from build123d import *

# Parameters (mm, degrees)
F0_W      = 28
F0_H      = 20
F1_DEPTH  = 20
F3_DEPTH  = 20
F6_DEPTH  = 17.5
F7_W      = 1.5
F7_H      = 4
F8_DEPTH  = 40
F12_DEPTH = 15
F15_D     = 14.5
F17_DEPTH = 20
F19_DEPTH = 12.5


with BuildPart() as f1:
    # F0 (on Top) → F1 (new body)
    with BuildSketch(Plane.XY):
        Rectangle(F0_W, F0_H)
    extrude(amount=F1_DEPTH)


with BuildPart() as f3:
    # F2 (on Top) → F3 (new body)
    with BuildSketch(Plane.XY):
        Polygon((-14, 3.5), (-7.5, 10), (-14, 10), align=None)
    extrude(amount=F3_DEPTH)


with BuildPart() as f4_1:
    # F4: instance of F3
    add(f3.part.mirror(Plane.YZ))


with BuildPart() as f6:
    # F5 (on Right) → F6 (new body, symmetric)
    with BuildSketch(Plane.YZ):
        Polygon((-4.741189, 25.532488), (10, 0), (10, 25.532488), align=None)
    extrude(amount=F6_DEPTH, both=True)


with BuildPart() as f8:
    # F7 (on Top) → F8 (new body)
    with BuildSketch(Plane.XY):
        with Locations((-13.25, 0)):
            Rectangle(F7_W, F7_H)
    extrude(amount=F8_DEPTH)


with BuildPart() as f9_1:
    # F9: instance of F8
    add(f8.part.mirror(Plane.YZ))


with BuildPart() as f1_1:
    add(f1.part)

    # F10: cut F3, F4_1, F6, F8, F9_1
    add(f3.part, mode=Mode.SUBTRACT)
    add(f4_1.part, mode=Mode.SUBTRACT)
    add(f6.part, mode=Mode.SUBTRACT)
    add(f8.part, mode=Mode.SUBTRACT)
    add(f9_1.part, mode=Mode.SUBTRACT)


with BuildPart() as f12:
    # F11 (on Right) → F12 (new body, symmetric)
    with BuildSketch(Plane.YZ):
        Polygon((-10, 24.094011), (-10, 1), (0, 6.773503), align=None)
    extrude(amount=F12_DEPTH, both=True)


with BuildPart() as f1_2:
    add(f1_1.part)

    # F13: cut F12
    add(f12.part, mode=Mode.SUBTRACT)

    # F15 (through all)
    with Locations(Plane(origin=(0, 2.933013, 1.693376), x_dir=(1, 0, 0), z_dir=(0, -0.866025, -0.5))):
        with Locations((0, 15.116025)):
            Hole(F15_D / 2)


with BuildPart() as f17:
    # F16 (on Right) → F17 (new body, symmetric)
    with BuildSketch(Plane.YZ):
        Polygon((-7.5, 13.205771), (6, 21), (-12, 21), align=None)
    extrude(amount=F17_DEPTH, both=True)


with BuildPart() as f19:
    # F18 (on face) → F19 (new body, symmetric)
    with BuildSketch(Plane(origin=(0, 7.5, 4.330127), x_dir=(-1, 0, 0), z_dir=(0, 0.866025, 0.5))):
        Polygon((14, 17.490759), (8, 17.490759), (14, 8), align=None)
    extrude(amount=F19_DEPTH, both=True)


with BuildPart() as f20_1:
    # F20: instance of F19
    add(f19.part.mirror(Plane.YZ))


with BuildPart() as f1_3:
    add(f1_2.part)

    # F21: cut F20_1, F19, F17
    add(f20_1.part, mode=Mode.SUBTRACT)
    add(f19.part, mode=Mode.SUBTRACT)
    add(f17.part, mode=Mode.SUBTRACT)


solid = f1_3.part
Verification items for the finished model (mm, model axes). A direction names the side the tool comes from. Coordinates: 2 decimals unless noted, no trailing zeros. Write each loop counter-clockwise with the first axis right and the second up, starting at its lowest first coordinate (ties: lowest second). Pieces come first, ordered by that corner, then holes. Notation, with made-up numbers: M 71,44 L 125,44 A17 ccw 125,74 Z; hole C -7,-39 d11. An arc over 180 degrees is marked long. One line per question, with ' | ' between items.
1) Sectioned sample at D-D on x = 5.5. Record the cut outline in (y, z).
Solutions:
outline: M -10,0 L 10,0 L 2.3,13.33 L -2.26,10.69 L 0,6.77 L -10,1 Z
2) Sectioned sample at B-B on z = 2.5. Record the cut outline in (x, y), then the cut area to 3 significant figures.
Solutions:
outline: M -14,-7.4 L 14,-7.4 L 14,-2 L 12.5,-2 L 12.5,2 L 14,2 L 14,3.5 L 8.94,8.56 L -8.94,8.56 L -14,3.5 L -14,2 L -12.5,2 L -12.5,-2 L -14,-2 Z | area: 409 mm^2
3) Depth check by flat-ended pin: pin 1 Ø1.5 at (y, z) = (7.5, 5) entering from +X; pin 2 Ø1 at (x, z) = (-10.5, 3.5) entering from +Y; pin 3 Ø8 at (x, y) = (10, 7.5) entering from +Z; pin 4 Ø4 at (y, z) = (-6, 4.5) entering from +X. Enter the tip coordinate at first touch or a pass-through.
Solutions:
pin 1: x = 10.75 | pin 2: y = 7.5 | pin 3: z = 11.26 | pin 4: x = 14
4) Material ranges on L1, parallel to X at y = 0.25, z = 1; L2, parallel to X at y = -2.25, z = 11.75; L3, parallel to Z at x = -8.5, y = -3.25, recorded low to high.
Solutions:
L1: -12.5 to 12.5 | L2: -11.91 to -6.16, 6.16 to 11.91 | L3: 0 to 4.9, 12.4 to 15.66
5) Sectioned sample at C-C on y = 6.5. Record the cut outline in (x, z), then the cut area to 3 significant figures.
Solutions:
outline: M -11,0 L 11,0 L 11,6.06 L -11,6.06 Z | area: 133 mm^2
6) Release check for a two-part mould opening along Y. For faces 5 (the face through (13, -2, 3)), 6 (the face through (14, 3, 6)), 7 (the face through (-11.5, 6, 4.3)) record: +Y half, -Y half, draft (parallel to the pull), parting line (faces both ways), or undercut.
Solutions:
face 5: undercut | face 6: draft | face 7: +Y half
7) Sectioned sample at A-A on x = -6. Record the cut outline in (y, z), then the cut area to 3 significant figures.
Solutions:
outline: M -10,0 L 10,0 L 1.98,13.9 L -2.59,11.26 L 0,6.77 L -10,1 Z | area: 129 mm^2
8) Access from +Z, -Z, +X, -X, +Y, -Y to the whole of each face (thin tool, end or side, straight path). Record for faces 1 (the face through (0.196, -5.07, 3.846)), 2 (the face through (-11.19, -0.97, 13.81)), 3 (the face through (-13, 2, 6)), 4 (the face through (13, 2, 6)).
Solutions:
face 1: +X, -X, -Y | face 2: +Z, -X, -Y | face 3: +Z, -Z, -X | face 4: +Z, -Z, +X
